Could you check a few things on this drawing? It's one solid part, dimensions in mm from its lowest x, y, z. Give positions to 0.01 mm unless a question says otherwise; leave off trailing zeros. Loops run counter-clockwise (first coordinate to the right, second up) from the corner with the lowest first, then second, coordinate; pieces in that order, holes last. Notation, with made-up numbers: M 35.25,17.5 L 60.25,17.5 A18 cw 60.25,29.5 Z; hole C 37,88.25 d2. An arc over 180 degrees is marked long. Answer as a JSON object with one key per item and string values.
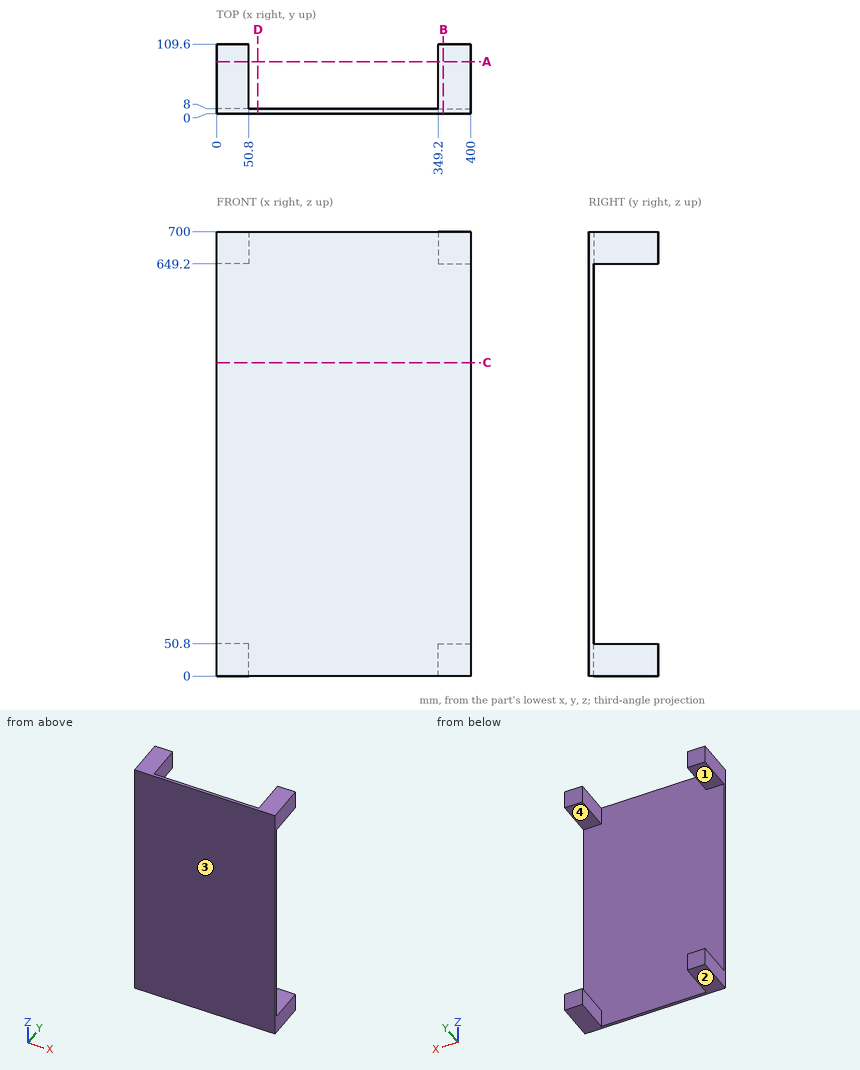
1) Suppose I cut it at D-D, the plane x = 65. Write out the boundary of the cut face in (y, z).
Answer list:
{"outline": "M 0,0 L 8,0 L 8,700 L 0,700 Z"}
2) If we mould it in two halves opening along Z, with no side actions, what happens to the marked faces 1, 2, 3 and 4? For each: +Z half, -Z half, draft (parallel to the pull), parting line (faces both ways), or undercut.
Answer list:
{"face 1": "undercut", "face 2": "-Z half", "face 3": "draft", "face 4": "undercut"}
3) Suppose I cut it at C-C, the plane z = 493.5. Write out the boundary of the cut face in (x, y).
Answer list:
{"outline": "M 0,0 L 400,0 L 400,8 L 0,8 Z"}
4) Suppose I cut it at A-A, the plane y = 82. Write out the boundary of the cut face in (x, z).
Answer list:
{"outline": "M 0,0 L 50.8,0 L 50.8,50.8 L 0,50.8 Z; M 0,649.2 L 50.8,649.2 L 50.8,700 L 0,700 Z; M 349.2,0 L 400,0 L 400,50.8 L 349.2,50.8 Z; M 349.2,649.2 L 400,649.2 L 400,700 L 349.2,700 Z"}
5) Suppose I cut it at B-B, the plane x = 357. Write out the boundary of the cut face in (y, z).
Answer list:
{"outline": "M 0,0 L 109.6,0 L 109.6,50.8 L 8,50.8 L 8,649.2 L 109.6,649.2 L 109.6,700 L 0,700 Z"}
6) Please list where these lines run through material, in increasing order: line 1 along Z through (x, y) = (384, 66); line 2 along Y through (x, z) = (183, 189). Write a range as from..to.
Answer list:
{"line 1": "0..50.8, 649.2..700", "line 2": "0..8"}
